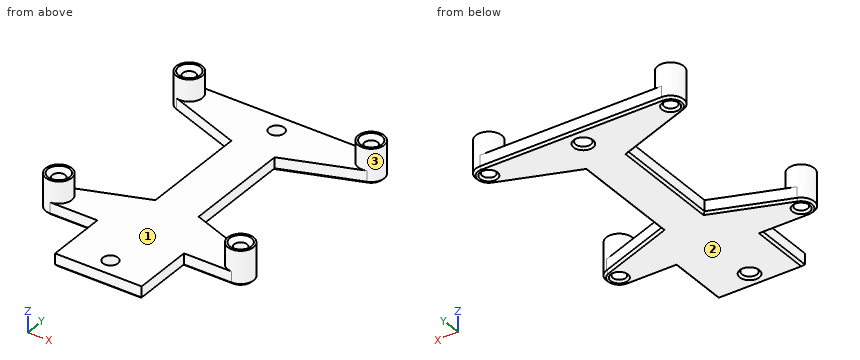
```python
from build123d import *

# Parameters (mm, degrees)
CYLINDER005_R     = 3
CYLINDER005_DEPTH = 8
PAD011_DEPTH      = 3
CYLINDER006_R     = 3
CYLINDER006_DEPTH = 8
SKETCH039_R       = 1.5
POCKET027_DEPTH   = 10
CHAMFER026_SIZE   = 1
SKETCH038_R       = 1.75
POCKET026_DEPTH   = 5
CHAMFER025_SIZE   = 0.5


with BuildPart() as keypadbracketscrewcylinder002:
    # Cylinder005 → Cylinder005 (new body)
    with BuildSketch(Plane(origin=(21, 13.5, 18), x_dir=(1, 0, 0), z_dir=(0, 0, 1))):
        Circle(CYLINDER005_R)
    extrude(amount=CYLINDER005_DEPTH)


with BuildPart() as keypadbracketpad008:
    # Sketch037 → Pad011 (new body)
    with BuildSketch(Plane.XY.offset(18)):
        with BuildLine():
            Line((0, -3.5), (10, -3.5))
            Line((10, -3.5), (10, 10.5))
            Line((10, 10.5), (21, 10.5))
            ThreePointArc((21, 10.5), (23.954423, 12.979055), (22.02606, 16.319078))
            Line((22.02606, 16.319078), (5, 22.516057))
            Line((5, 22.516057), (5, 47.663943))
            Line((5, 47.663943), (22.02606, 53.860922))
            ThreePointArc((22.02606, 53.860922), (23.954423, 57.200945), (21, 59.68))
            Line((21, 59.68), (0, 59.68))
            Line((0, 59.68), (0, -3.5))
        make_face()
    extrude(amount=PAD011_DEPTH)


with BuildPart() as keypadbracketscrewholeschamfer019:
    # Cylinder006 → Cylinder006 (new body)
    with BuildSketch(Plane(origin=(21, 56.68, 18), x_dir=(1, 0, 0), z_dir=(0, 0, 1))):
        Circle(CYLINDER006_R)
    extrude(amount=CYLINDER006_DEPTH)

    # Fusion005: union KeypadBracketScrewCylinder002, KeypadBracketPad008
    add(keypadbracketscrewcylinder002.part)
    add(keypadbracketpad008.part)

    # Sketch039 → Pocket027 (cut)
    with BuildSketch(Plane.XY.offset(26)):
        with Locations((21, 13.5)):
            Circle(SKETCH039_R)
        with Locations((21, 56.68)):
            Circle(SKETCH039_R)
    extrude(amount=-POCKET027_DEPTH, mode=Mode.SUBTRACT)

    # Chamfer026
    chamfer026_edges = [keypadbracketscrewholeschamfer019.edges().sort_by_distance(p)[0] for p in [
        (19.5, 56.68, 26),
        (19.5, 13.5, 26),
    ]]
    chamfer(chamfer026_edges, length=CHAMFER026_SIZE)


with BuildPart() as keypadbracketprintingchamfer019_final001:
    # Part__Mirroring005: instance of KeypadBracketScrewHolesChamfer019
    add(keypadbracketscrewholeschamfer019.part.mirror(Plane(origin=(0, 0, 0), x_dir=(0, -1, 0), z_dir=(1, 0, 0))))

    # Fusion006: union KeypadBracketScrewHolesChamfer019
    add(keypadbracketscrewholeschamfer019.part)

    # Sketch038 → Pocket026 (cut)
    with BuildSketch(Plane.XY.offset(21)):
        with Locations((0, 0.5)):
            Circle(SKETCH038_R)
        with Locations((0, 55.5)):
            Circle(SKETCH038_R)
    extrude(amount=-POCKET026_DEPTH, mode=Mode.SUBTRACT)

    # Chamfer025
    chamfer025_edges = [keypadbracketprintingchamfer019_final001.edges().sort_by_distance(p)[0] for p in [
        (-21, 15, 18),
        (-21, 12, 18),
        (0, 57.25, 18),
        (0, 53.75, 18),
        (0, 2.25, 18),
        (0, -1.25, 18),
        (-23.12132, 58.80132, 18),
        (-23.457456, 54.959271, 18),
        (0, 59.68, 18),
        (-13.51303, 50.762433, 18),
        (23.12132, 58.80132, 18),
        (-5, 35.09, 18),
        (23.457456, 54.959271, 18),
        (-13.51303, 19.417567, 18),
        (13.51303, 50.762433, 18),
        (-23.457456, 15.220729, 18),
        (5, 35.09, 18),
        (-23.12132, 11.37868, 18),
        (13.51303, 19.417567, 18),
        (-15.5, 10.5, 18),
        (23.457456, 15.220729, 18),
        (-10, 3.5, 18),
        (23.12132, 11.37868, 18),
        (0, -3.5, 18),
        (15.5, 10.5, 18),
        (10, 3.5, 18),
        (-21, 58.18, 18),
        (-21, 55.18, 18),
        (21, 58.18, 18),
        (21, 55.18, 18),
        (21, 15, 18),
        (21, 12, 18),
    ]]
    chamfer(chamfer025_edges, length=CHAMFER025_SIZE)


solid = keypadbracketprintingchamfer019_final001.part
```
Source: CAD feature listing. Evaluate the final solid. Frame: model axes, mm. Face numbers are marked on the shaded views. Round coordinates to 2 decimals unless told otherwise and drop trailing zeros. Order: outer loops, then holes, each group sorted by start corner. A loop starts at its lowest first (then second) coordinate and runs counter-clockwise, first axis right, second up. Notation, with made-up numbers: (35.25, -30.5) -> (50.25, -30.5) arc R29 cw to (50.25, -6.5) -> close; hole circle Ø4 at (80, -12). An arc over 180 degrees is marked (long way). Use CSV: the item, a comma, the result in double quotes.
(1) Pull-direction query (X, two-part tool) for the marked faces 1, 2 and 3; classes: +X half, -X half, draft (parallel to the pull), parting line (faces both ways), or undercut.
Report:
face 1,"undercut"
face 2,"draft"
face 3,"undercut"
(2) Section D-D on x = 16. Return the cut outline in (y, z), and give its area (3 significant figures).
Report:
outline,"(10.5, 18.5) -> (11, 18) -> (17.98, 18) -> (18.51, 18.5) -> (18.51, 21) -> (10.5, 21) -> close; (51.67, 18.5) -> (52.2, 18) -> (59.18, 18) -> (59.68, 18.5) -> (59.68, 21) -> (51.67, 21) -> close"
area,"47.6 mm^2"
(3) Section C-C on y = 0.5. Return the cut outline in (x, z), and give its area (3 significant figures).
Report:
outline,"(-10, 18.5) -> (-9.5, 18) -> (-2.25, 18) -> (-1.75, 18.5) -> (-1.75, 21) -> (-10, 21) -> close; (1.75, 18.5) -> (2.25, 18) -> (9.5, 18) -> (10, 18.5) -> (10, 21) -> (1.75, 21) -> close"
area,"49.0 mm^2"
(4) Ray query, L1, parallel to Y at x = 21, z = 22; L2, parallel to Y at x = 0, z = 20.05; L3, parallel to Z at x = -4, y = 49.5. Return the intervals inside material, ascending.
Report:
L1,"10.5 to 12, 15 to 16.5, 53.68 to 55.18, 58.18 to 59.68"
L2,"-3.5 to -1.25, 2.25 to 53.75, 57.25 to 59.68"
L3,"18 to 21"
(5) First-contact query: pin 1 Ø4 at (x, y) = (-0.5, 35.5) entering from +Z; pin 2 Ø3.5 at (x, y) = (21, 56.68) entering from +Z; pin 3 Ø2 at (x, z) = (13.5, 20) entering from -Y; pin 4 Ø3 at (y, z) = (12.5, 23) entering from -X. Flat tips, straight axial feed; report the tip coordinate or a pass-through.
Report:
pin 1,"z = 21"
pin 2,"z = 25.25"
pin 3,"y = 10.5"
pin 4,"x = -24"
(6) Section B-B on x = 0. Return the cut outline in (y, z).
Report:
outline,"(-3.5, 18.5) -> (-3, 18) -> (-1.75, 18) -> (-1.25, 18.5) -> (-1.25, 21) -> (-3.5, 21) -> close; (2.25, 18.5) -> (2.75, 18) -> (53.25, 18) -> (53.75, 18.5) -> (53.75, 21) -> (2.25, 21) -> close; (57.25, 18.5) -> (57.75, 18) -> (59.18, 18) -> (59.68, 18.5) -> (59.68, 21) -> (57.25, 21) -> close"
(7) Section A-A on z = 23. Return the cut outline in (x, y), and give its area (3 significant figures).
Report:
outline,"circle Ø6 at (-21, 13.5); circle Ø6 at (-21, 56.68); circle Ø6 at (21, 13.5); circle Ø6 at (21, 56.68); hole circle Ø3 at (-21, 13.5); hole circle Ø3 at (-21, 56.68); hole circle Ø3 at (21, 13.5); hole circle Ø3 at (21, 56.68)"
area,"84.8 mm^2"
